Read the model definition and answer for the solid it produces. Units are mm, in the model's axes. A direction names the side the tool comes from. Round coordinates to 2 decimals unless told otherwise and drop trailing zeros. Order: outer loops, then holes, each group sorted by start corner. A loop starts at its lowest first (then second) coordinate and runs counter-clockwise, first axis right, second up. Notation, with made-up numbers: (-10.75, 7) -> (11.25, 7) arc R24 cw to (11.25, 39) -> close; hole circle Ø11 at (9.5, 31). An arc over 180 degrees is marked (long way). Answer as a JSON object with one key per item and string values. Group by question number.
Item 1: Section B-B, the plane x = -14 is taken. Write down the section's boundary in (y, z), plus the area to 3 significant figures.
Item 2: Given P1, Ø2, axis at x = 20, z = 3, coming from the +Y side; P2, Ø1.5, axis at y = 7.5, z = 3, coming from the +X side, each flat-ended and moving along its own axis, determine where each tip first touches the part or whether it passes through.
Item 3: Section C-C, the plane y = 18 is taken. Write down the section's boundary in (x, z).
Item 4: The mould has two halves that part along X. Classify faces 6 (the flat face through (23, -25, 3)), 7 (the flat face through (30, 0, 3)), 8 (the flat face through (-20, 15, 3)), 9 (the flat face through (-30, -14, 3)): pulls with the +X half, pulls with the -X half, needs draft (parallel to the pull), parting line crosses it, or undercut.
Item 5: Consider probe 1 along Y at (x, z) = (14, 4.55); probe 2 along X at (y, z) = (15.5, 1.5); probe 3 along X at (y, z) = (22.5, 3). Determine where each line is inside the solid, lowest interval first. Write a range as from..to.
Item 6: Section A-A, the plane y = 0 is taken. Write down the section's boundary in (x, z), plus the area to 3 significant figures.
Item 7: Section D-D, the plane y = -10 is taken. Write down the section's boundary in (x, z), plus the area to 3 significant figures.
Item 8: For faces 1 (the cylindrical face through (-18.81, -20.07, 3.38)), 2 (the cylindrical face through (25.07, 7.021, 1.845)), 3 (the cylindrical face through (-25.07, 7.021, 4.155)), 4 (the cylindrical face through (-11.6, -13, 3)), 5 (the cylindrical face through (-0.16, 20.07, 1.76)), determine the directions among +Z, -Z, +X, -X, +Y, -Y from which every point of the face is accessible in a straight line to the end or side of a thin tool.
Autodesk Inventor part; units mm, degrees
ref_plane "YZ Plane" through (0, 0, 0) normal (1, 0, 0) x (0, 1, 0)
ref_plane "XZ Plane" through (0, 0, 0) normal (0, 1, 0) x (-1, 0, 0)
ref_plane "XY Plane" through (0, 0, 0) normal (0, 0, 1) x (1, 0, 0)
sketch "スケッチ1" plane through (0, 0, 0) normal (0, 0, 1) x (1, 0, 0)
  circle A0 centre (0, 0) radius 13
  circle A1 centre (-14, 14) radius 2.6
  circle A2 centre (14, 14) radius 2.6
  circle A3 centre (14, -14) radius 2.6
  circle A4 centre (-14, -14) radius 2.6
  line L0 (25, 25) -> (20.5385, 25)
  line L1 (-30, 20) -> (-30, 8.0385)
  line L2 (-25, -25) -> (-20.5385, -25)
  line L3 (30, -20) -> (30, -8.0385)
  line L4 (30, 25) -> (-30, -25) construction
  line L5 (-30, 25) -> (30, -25) construction
  arc A5 (-19.4615, 25) -> (-20.5385, 25) centre (-20, 26.4) ccw construction
  arc A6 (0.5385, 25) -> (-0.5385, 25) centre (0, 26.4) ccw construction
  arc A7 (20.5385, 25) -> (19.4615, 25) centre (20, 26.4) ccw construction
  arc A8 (-20.5385, 25) -> (-19.4615, 25) centre (-20, 26.4) ccw
  line L6 (-19.4615, 25) -> (-20.5385, 25) construction
  line L7 (-20.5385, 25) -> (-25, 25)
  arc A9 (-0.5385, 25) -> (0.5385, 25) centre (0, 26.4) ccw
  line L8 (0.5385, 25) -> (-0.5385, 25) construction
  line L9 (-0.5385, 25) -> (-19.4615, 25)
  arc A10 (19.4615, 25) -> (20.5385, 25) centre (20, 26.4) ccw
  line L10 (20.5385, 25) -> (19.4615, 25) construction
  line L11 (19.4615, 25) -> (0.5385, 25)
  arc A11 (-0.5385, -25) -> (0.5385, -25) centre (0, -26.4) ccw construction
  arc A12 (-20.5385, -25) -> (-19.4615, -25) centre (-20, -26.4) ccw construction
  arc A13 (19.4615, -25) -> (20.5385, -25) centre (20, -26.4) ccw construction
  arc A14 (-19.4615, -25) -> (-20.5385, -25) centre (-20, -26.4) ccw
  line L12 (-19.4615, -25) -> (-0.5385, -25)
  line L13 (-20.5385, -25) -> (-19.4615, -25) construction
  arc A15 (0.5385, -25) -> (-0.5385, -25) centre (0, -26.4) ccw
  line L14 (0.5385, -25) -> (19.4615, -25)
  line L15 (-0.5385, -25) -> (0.5385, -25) construction
  arc A16 (20.5385, -25) -> (19.4615, -25) centre (20, -26.4) ccw
  line L16 (20.5385, -25) -> (25, -25)
  line L17 (19.4615, -25) -> (20.5385, -25) construction
  arc A17 (-30, 8.0385) -> (-30, 6.9615) centre (-31.4, 7.5) ccw construction
  arc A18 (-30, -6.9615) -> (-30, -8.0385) centre (-31.4, -7.5) ccw construction
  arc A19 (30, 6.9615) -> (30, 8.0385) centre (31.4, 7.5) ccw construction
  arc A20 (30, -8.0385) -> (30, -6.9615) centre (31.4, -7.5) ccw construction
  arc A21 (-30, 6.9615) -> (-30, 8.0385) centre (-31.4, 7.5) ccw
  line L18 (-30, 6.9615) -> (-30, -6.9615)
  line L19 (-30, 8.0385) -> (-30, 6.9615) construction
  arc A22 (-30, -8.0385) -> (-30, -6.9615) centre (-31.4, -7.5) ccw
  line L20 (-30, -8.0385) -> (-30, -20)
  line L21 (-30, -6.9615) -> (-30, -8.0385) construction
  arc A23 (30, 8.0385) -> (30, 6.9615) centre (31.4, 7.5) ccw
  line L22 (30, 6.9615) -> (30, 8.0385) construction
  line L23 (30, 8.0385) -> (30, 20)
  arc A24 (30, -6.9615) -> (30, -8.0385) centre (31.4, -7.5) ccw
  line L24 (30, -6.9615) -> (30, 6.9615)
  line L25 (30, -8.0385) -> (30, -6.9615) construction
  arc A25 (-25, 25) -> (-30, 20) centre (-25, 20) ccw
  arc A26 (30, 20) -> (25, 25) centre (25, 20) ccw
  arc A27 (25, -25) -> (30, -20) centre (25, -20) ccw
  arc A28 (-30, -20) -> (-25, -25) centre (-25, -20) ccw
  point P0 (0, 0)
  point P1 (0, 0)
  dimension "d0" = 26
  dimension "d1" = 28
  dimension "d2" = 14
  dimension "d3" = 5.2
  dimension "d4" = 5.2
  dimension "d5" = 28
  dimension "d6" = 14
  dimension "d7" = 5.2
  dimension "d8" = 5.2
  dimension "d9" = 60
  dimension "d10" = 50
  dimension "d11" = 3
  dimension "d12" = 3
  dimension "d13" = 20
  dimension "d14" = 3
  dimension "d15" = 20
  dimension "d16" = 1.4
  dimension "d17" = 3
  dimension "d18" = 3
  dimension "d19" = 3
  dimension "d20" = 20
  dimension "d21" = 20
  dimension "d22" = 1.4
  dimension "d23" = 3
  dimension "d24" = 3
  dimension "d25" = 3
  dimension "d26" = 3
  dimension "d27" = 15
  dimension "d28" = 15
  dimension "d29" = 7.5
  dimension "d30" = 7.5
  dimension "d31" = 1.4
  dimension "d32" = 1.4
  dimension "d33" = 5
extrude "押し出し1" add sketch "スケッチ1" along normal blind 6
sketch "スケッチ2" plane through (-19.4615, 25, 0) normal (0, 1, 0) x (1, 0, 0)
  circle A0 centre (-0.5385, -3) radius 1.25
  circle A1 centre (19.4615, -3) radius 1.25
  circle A2 centre (39.4615, -3) radius 1.25
  point P0 (19.4615, 0)
  dimension "d36" = 2.5
  dimension "d37" = 2.5
  dimension "d38" = 2.5
  dimension "d39" = 3
  dimension "d40" = 20
  dimension "d41" = 20
sketch "スケッチ3" plane through (30, -6.9615, 0) normal (1, 0, 0) x (0, 0, -1)
  circle A0 centre (-3, 14.4615) radius 1.25
  circle A1 centre (-3, -0.5385) radius 1.25
  point P0 (0, 6.9615)
  dimension "d42" = 2.5
  dimension "d43" = 2.5
  dimension "d44" = 3
  dimension "d45" = 7.5
  dimension "d46" = 7.5
extrude "押し出し2" cut sketch "スケッチ3" against normal blind 10
extrude "押し出し3" cut sketch "スケッチ2" against normal blind 10
sketch "スケッチ4" plane through (0.5385, -25, 0) normal (0, -1, 0) x (1, 0, 0)
  circle A0 centre (-0.5385, 3) radius 1.25
  circle A1 centre (-20.5385, 3) radius 1.25
  circle A2 centre (19.4615, 3) radius 1.25
  point P0 (-0.5385, 0)
  dimension "d51" = 2.5
  dimension "d52" = 2.5
  dimension "d53" = 2.5
  dimension "d54" = 20
  dimension "d55" = 20
  dimension "d56" = 3
extrude "押し出し4" cut sketch "スケッチ4" against normal blind 10
sketch "スケッチ5" plane through (-30, -6.9615, 0) normal (-1, 0, 0) x (0, 0, 1)
  circle A0 centre (3, 14.4615) radius 1.25
  circle A1 centre (3, -0.5385) radius 1.25
  point P0 (0, 6.9615)
extrude "押し出し5" cut sketch "スケッチ5" against normal blind 10
equation "\"d29\" = 0.5 * d27"
properties part number "エアシリンダマウント" material "ポリカーボネート、スモーク"
Values found:
{
 "1": {"outline": "(-25, 0) -> (-16.6, 0) -> (-16.6, 6) -> (-25, 6) -> close; (-11.4, 0) -> (11.4, 0) -> (11.4, 6) -> (-11.4, 6) -> close; (16.6, 0) -> (25, 0) -> (25, 6) -> (16.6, 6) -> close", "area": "238 mm2"},
 "2": {"P1": "y = 15", "P2": "x = 20"},
 "3": {"outline": "(-30, 0) -> (30, 0) -> (30, 6) -> (-30, 6) -> close; hole circle Ø2.5 at (-20, 3); hole circle Ø2.5 at (0, 3); hole circle Ø2.5 at (20, 3)"},
 "4": {"face 6": "needs draft", "face 7": "pulls with the +X half", "face 8": "undercut", "face 9": "pulls with the -X half"},
 "5": {"probe 1": "-25..-16.6, -11.4..11.4, 16.6..25", "probe 2": "-30..-16.12, -11.88..11.88, 16.12..30", "probe 3": "-29.33..-21.25, -18.75..-1.25, 1.25..18.75, 21.25..29.33"},
 "6": {"outline": "(-30, 0) -> (-13, 0) -> (-13, 6) -> (-30, 6) -> close; (13, 0) -> (30, 0) -> (30, 6) -> (13, 6) -> close", "area": "204 mm2"},
 "7": {"outline": "(-30, 0) -> (-8.31, 0) -> (-8.31, 6) -> (-30, 6) -> close; (8.31, 0) -> (30, 0) -> (30, 6) -> (8.31, 6) -> close", "area": "260 mm2"},
 "8": {"face 1": "-Y", "face 2": "+X", "face 3": "-X", "face 4": "+Z, -Z", "face 5": "+Y"}
}
